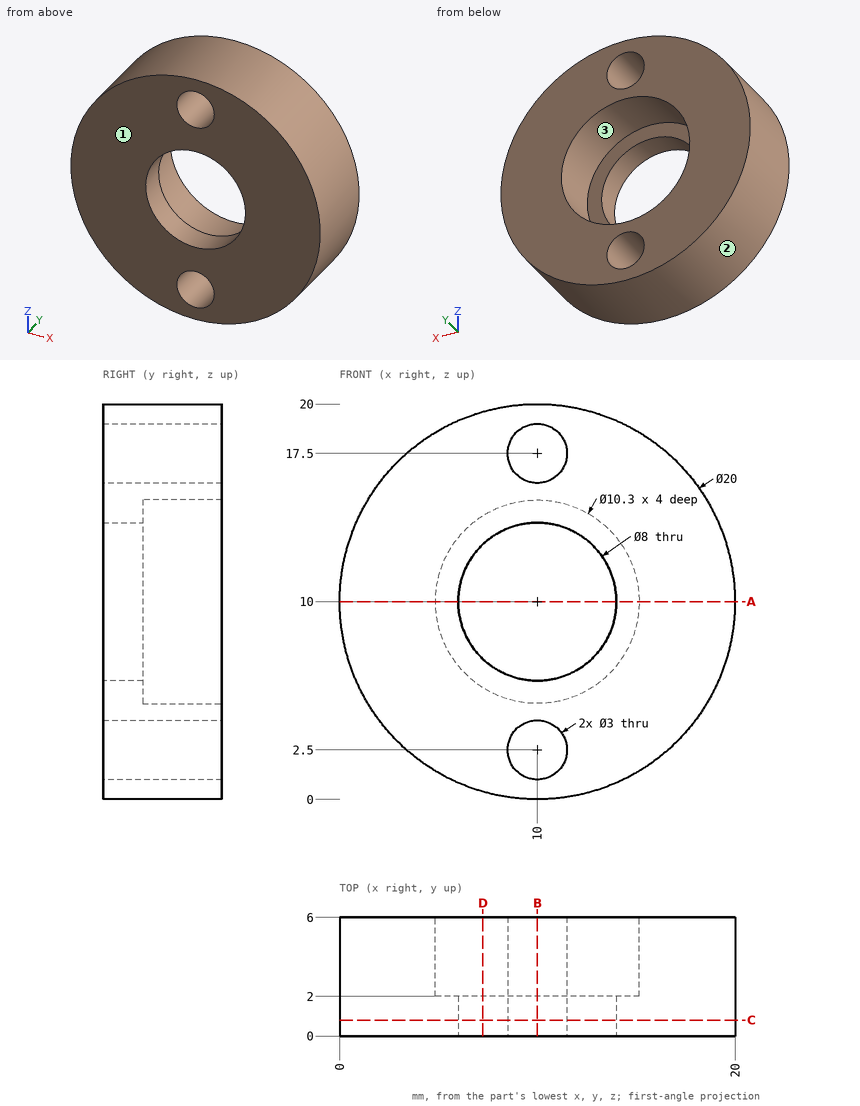
Answer from the drawing. Dimensions are ordinates in mm from the lowest x, y and z of the part. Coordinates: 2 decimals unless noted, no trailing zeros. Write each loop counter-clockwise with the first axis right and the second up, starting at its lowest first coordinate (ties: lowest second). Pieces come first, ordered by that corner, then holes. Notation, with made-up numbers: M 1.25,5 L 42.25,5 A18 cw 42.25,17 Z; hole C -36.75,6 d4. An arc over 180 degrees is marked long. Use a Markdown table: item, result.
Q1. The part is cut by section B-B, the plane x = 10. Write down the section's boundary in (y, z), then the cut area to 3 significant figures.
Answer block:
| item | result |
|---|---|
| outline | M 0,0 L 6,0 L 6,1 L 0,1 Z; M 0,4 L 6,4 L 6,4.85 L 2,4.85 L 2,6 L 0,6 Z; M 0,14 L 2,14 L 2,15.15 L 6,15.15 L 6,16 L 0,16 Z; M 0,19 L 6,19 L 6,20 L 0,20 Z |
| area | 26.8 mm2 |
Q2. The part is cut by section C-C, the plane y = 0.8. Write down the section's boundary in (x, z).
Answer block:
| item | result |
|---|---|
| outline | C 10,10 d20; hole C 10,10 d8; hole C 10,2.5 d3; hole C 10,17.5 d3 |
Q3. Determine the mould class of the marked faces 1, 2 and 3 for opening direction X: released by +X, released by -X, zero draft, split by the parting line, or undercut.
Answer block:
| item | result |
|---|---|
| face 1 | zero draft |
| face 2 | split by the parting line |
| face 3 | undercut |
Q4. Straight lines are drawn through the part: L1, parallel to X at y = 1.65, z = 10; L2, parallel to Z at x = 10.5, y = 5.6; L3, parallel to X at y = 5.5, z = 8. For each, find the intervals that lie inside material, in ascending order. Write a range as [from, to].
Answer block:
| item | result |
|---|---|
| L1 | x = [0, 6], [14, 20] |
| L2 | z = [0.01, 1.09], [3.91, 4.87], [15.13, 16.09], [18.91, 19.99] |
| L3 | x = [0.2, 5.25], [14.75, 19.8] |
Q5. The part is cut by section A-A, the plane z = 10. Write down the section's boundary in (x, y).
Answer block:
| item | result |
|---|---|
| outline | M 0,0 L 6,0 L 6,2 L 4.85,2 L 4.85,6 L 0,6 Z; M 14,0 L 20,0 L 20,6 L 15.15,6 L 15.15,2 L 14,2 Z |
Q6. The part is cut by section D-D, the plane x = 7.25. Write down the section's boundary in (y, z), then the cut area to 3 significant figures.
Answer block:
| item | result |
|---|---|
| outline | M 0,0.39 L 6,0.39 L 6,5.65 L 2,5.65 L 2,7.1 L 0,7.1 Z; M 0,12.9 L 2,12.9 L 2,14.35 L 6,14.35 L 6,19.61 L 0,19.61 Z |
| area | 68.9 mm2 |
Q7. Each of these flat-tipped pins is pushed along its axis until it touches: pin 1 Ø3 at (y, z) = (3.5, 5) entering from +X; pin 2 Ø1 at (y, z) = (3, 7) entering from +X; pin 3 Ø1.5 at (y, z) = (3.5, 4.5) entering from +X. Where does it stop, or does it pass through?
Answer block:
| item | result |
|---|---|
| pin 1 | stops at x = 19.37 |
| pin 2 | stops at x = 19.68 |
| pin 3 | stops at x = 18.8 |
